Geometry check sheet. Reference: drawing and pictorial views, mm from the part's lowest x, y, z. A direction names the side the tool comes from. Round coordinates to 2 decimals unless told otherwise and drop trailing zeros. Order: outer loops, then holes, each group sorted by start corner. A loop starts at its lowest first (then second) coordinate and runs counter-clockwise, first axis right, second up. Notation, with made-up numbers: (39, 49) -> (67, 49) arc R25 cw to (67, 84) -> close; hole circle Ø8 at (35.25, 35.25). An arc over 180 degrees is marked (long way). Put each result on its own line as item: value.
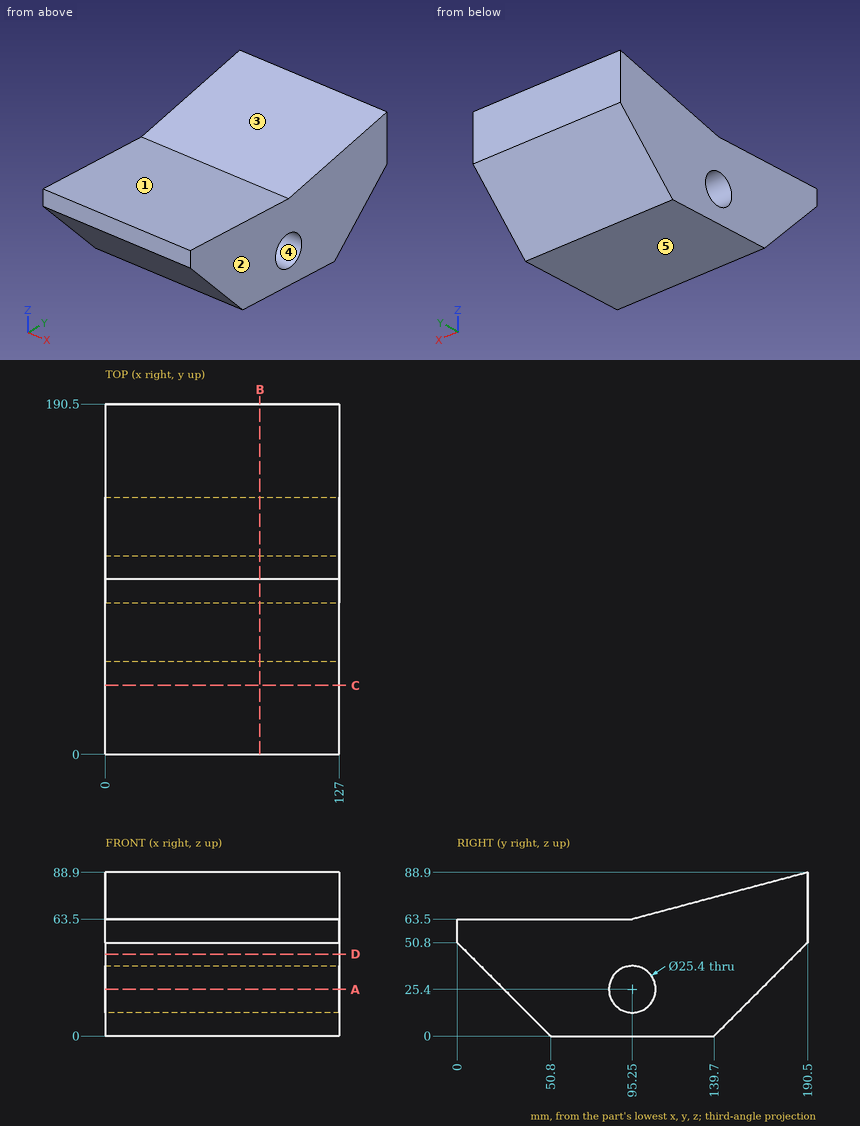
Item 1: Release check for a two-part mould opening along Y. For the marked faces 3, 4 and 5 record: pulls with the +Y half, pulls with the -Y half, needs draft (parallel to the pull), parting line crosses it, or undercut.
Geometry check:
face 3: pulls with the -Y half
face 4: undercut
face 5: needs draft
Item 2: Sectioned sample at A-A, the plane z = 25.4. Record the boundary of the cut face in (x, y).
Geometry check:
outline: (0, 25.4) -> (127, 25.4) -> (127, 82.55) -> (0, 82.55) -> close; (0, 107.95) -> (127, 107.95) -> (127, 165.1) -> (0, 165.1) -> close
Item 3: Depth check by flat-ended pin: pin 1 Ø4 at (x, z) = (101.5, 50) entering from +Y; pin 2 Ø5 at (x, z) = (49, 47.5) entering from -Y; pin 3 Ø10 at (x, z) = (59.5, 31.5) entering from -Y; pin 4 Ø5 at (x, y) = (79.5, 40) entering from +Z. Enter the tip coordinate at first touch or a pass-through.
Geometry check:
pin 1: y = 190.5
pin 2: y = 0.8
pin 3: y = 14.3
pin 4: z = 63.5
Item 4: Sectioned sample at C-C, the plane y = 37.5. Record the boundary of the cut face in (x, z), then the cut area to 3 significant figures.
Geometry check:
outline: (0, 13.3) -> (127, 13.3) -> (127, 63.5) -> (0, 63.5) -> close
area: 6,380 mm2
Item 5: Tool access check on the marked faces 1 and 2. Record the directions out of +Z, -Z, +X, -X, +Y, -Y that give a thin tool (end or side, any length) a straight path to the whole face; none if there is none.
Geometry check:
face 1: +Z, +X, -X, -Y
face 2: +Z, -Z, +X, +Y, -Y
Item 6: Sectioned sample at D-D, the plane z = 44.5. Record the boundary of the cut face in (x, y).
Geometry check:
outline: (0, 6.3) -> (127, 6.3) -> (127, 184.2) -> (0, 184.2) -> close
Item 7: Material ranges on line 1 along Z through (x, y) = (35, 95); line 2 along Z through (x, y) = (118, 66); line 3 along Y through (x, z) = (96, 25), recorded low to high.
Geometry check:
line 1: 0 to 12.7, 38.1 to 63.5
line 2: 0 to 63.5
line 3: 25.8 to 82.56, 107.94 to 164.7
Item 8: Sectioned sample at B-B, the plane x = 84. Record the boundary of the cut face in (y, z).
Geometry check:
outline: (0, 50.8) -> (50.8, 0) -> (139.7, 0) -> (190.5, 50.8) -> (190.5, 88.9) -> (95.25, 63.5) -> (0, 63.5) -> close; hole circle Ø25.4 at (95.25, 25.4)
